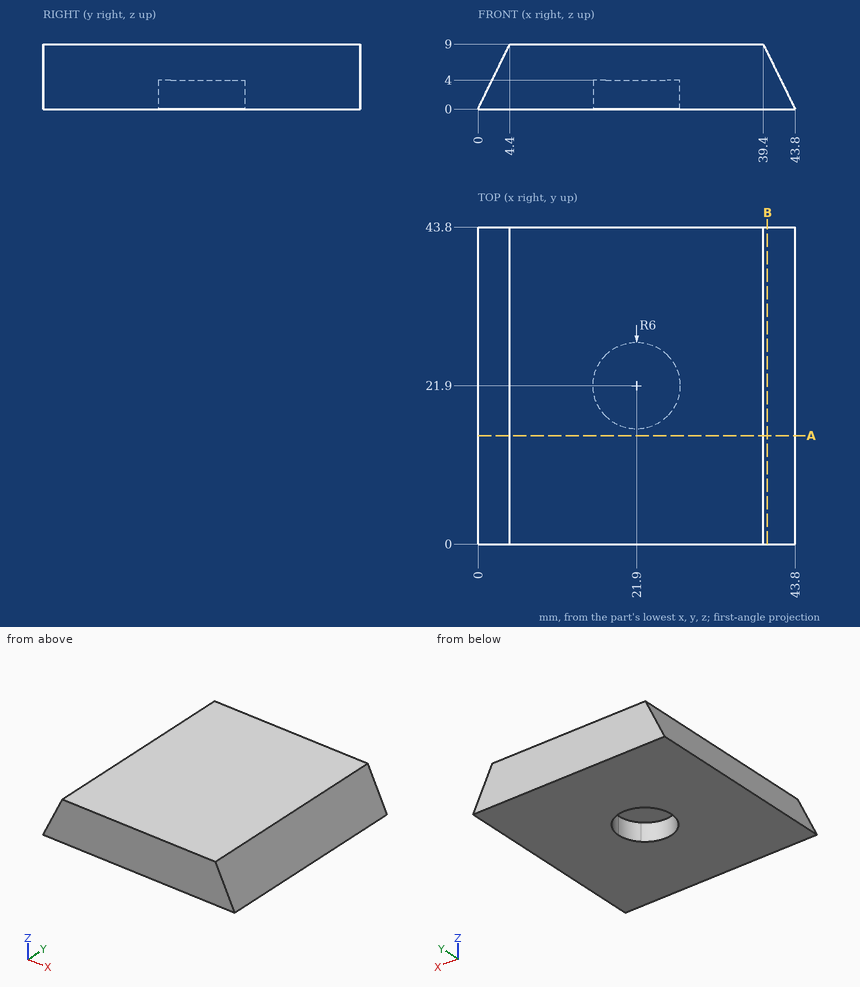
For this review, use the dimensioned drawing (mm, ordinates from the lowest corner) and the shaded views. Give positions to 0.01 mm unless a question says otherwise; leave off trailing zeros. Write each loop counter-clockwise with the first axis right and the second up, starting at its lowest first coordinate (ties: lowest second). Pieces come first, ordered by that corner, then holes. Notation, with made-up numbers: M 71,-7 L 94,-7 A24 ccw 94,17 Z; hole C 37.5,36.5 d10. An arc over 180 degrees is marked long. Write item = value, one per line. Start each with the question number.
Q1. Clearance check with flat-ended pins moving along their axes: pin 1 (1 mm diameter, centred on y = 15.5, z = 2.5, fed in from -X); pin 2 (1.5 mm diameter, centred on y = 39, z = 2.5, fed in from -X); pin 3 (1 mm diameter, centred on x = 23, y = 20, fed in from -Z). State where each tip first meets the part, or that it passes through.
Q2. We need section A-A (y = 15). State the section outline as (x, z) points, plus the area to 3 significant figures.
Q3. We need section B-B (x = 40). State the section outline as (y, z) points, plus the area to 3 significant figures.
Q4. For line 1 (X direction, y = 23.5, z = 3.75); line 2 (Y direction, x = 23, z = 1.25); line 3 (X direction, y = 22.5, z = 3), list the stretches that pass through material, from the lowest coordinate up.
Result set:
q1.pin_1 = 0.98
q1.pin_2 = 0.86
q1.pin_3 = 4
q2.outline = M 0,0 L 43.8,0 L 39.4,9 L 4.4,9 Z
q2.area = 355 mm2
q3.outline = M 0,0 L 43.8,0 L 43.8,7.77 L 0,7.77 Z
q3.area = 340 mm2
q4.line_1 = 1.83 to 16.12, 27.68 to 41.97
q4.line_2 = 0 to 16, 27.8 to 43.8
q4.line_3 = 1.47 to 15.93, 27.87 to 42.33
